from build123d import *

# Parameters (mm, degrees)
SKETCH_1_R      = 2.5
EXTRUDE_1_DEPTH = 4
FILLET_1_R      = 5


with BuildPart() as part:
    # ｽｹｯﾁ1 → ﾎﾞｽ - 押し出し1 (new body)
    with BuildSketch(Plane.XY):
        Polygon((0, 15), (0, 0), (4, 0), (4, -6), (8.110763801, -6), (24, -2.18322685), (24, 8.312378031), (4, 22), (4, 15), align=None)
        with Locations((14, 3)):
            Circle(SKETCH_1_R, mode=Mode.SUBTRACT)
    extrude(amount=EXTRUDE_1_DEPTH)

    # ﾌｨﾚｯﾄ1
    fillet_1_edges = [part.edges().sort_by_distance(p)[0] for p in [
        (24, -2.18322685, 2),
        (24, 8.312378031, 2),
    ]]
    fillet(fillet_1_edges, radius=FILLET_1_R)


solid = part.part
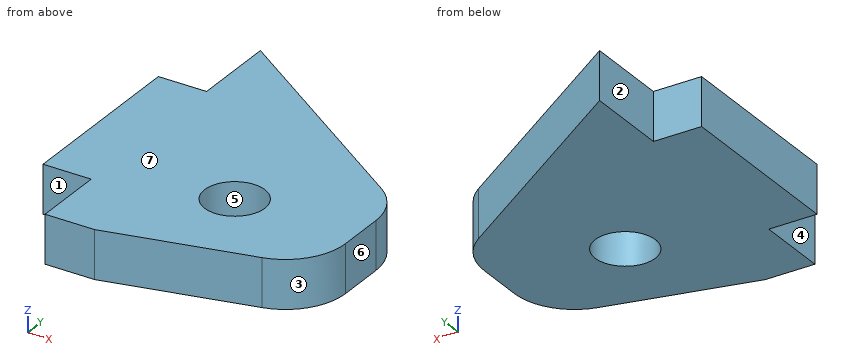
Read the model definition and answer for the solid it produces. Units are mm, in the model's axes. Face numbers are marked on the shaded views. A direction names the side the tool comes from. Give positions to 0.01 mm unless a question says otherwise; leave off trailing zeros. Write each loop counter-clockwise with the first axis right and the second up, starting at its lowest first coordinate (ties: lowest second). Pieces come first, ordered by that corner, then holes. Notation, with made-up numbers: M 2.5,7 L 47.5,7 A30 ccw 47.5,41 Z; hole C 67.25,-34.5 d11. An arc over 180 degrees is marked long. One line per item, written item: value. Start each with the question number.
(1) Find section A-A (z = 3.7). Determine the outline of the cut face in (x, y), plus the area to 3 significant figures.
(2) Find section D-D (x = 2.25). Determine the outline of the cut face in (y, z).
(3) Find section C-C (x = 13.5). Determine the outline of the cut face in (y, z).
(4) A tool of negligible diameter and unlimited length cuts with its end or side. For the marked faces 1, 2 and 3, from which of +Z, -Z, +X, -X, +Y, -Y can it reach the whole face along a straight path? Write none if from no direction.
(5) Flat-ended cylindrical pins translate along their axes: pin 1 Ø1.2 at (y, z) = (17.5, 2.5) entering from -X; pin 2 Ø3 at (x, y) = (14, 3) entering from -Z; pin 3 Ø2 at (x, z) = (8.5, 2.5) entering from +Y. Find the tip coordinate at first contact, or state that the pin passes through.
(6) Find the intervals of material crossed by line 1 (X direction, y = 2.5, z = 0.25); line 2 (X direction, y = 2.75, z = 3.5); line 3 (Y direction, x = 3.75, z = 3.55), in increasing order.
(7) Determine the mould class of the marked faces 4, 5, 6 and 7 for opening direction X: pulls with the +X half, pulls with the -X half, needs draft (parallel to the pull), parting line crosses it, or undercut.
(8) Find section B-B (y = 3). Determine the outline of the cut face in (x, z).
Results below:
1. outline: M 0,0 L 4,0 L 4,-6 L 8.11,-6 L 20.17,-3.1 A5 ccw 24,1.76 L 24,5.68 A5 ccw 21.82,9.8 L 4,22 L 4,15 L 0,15 Z; hole C 14,3 d5
1. area: 429 mm^2
2. outline: M 0,0 L 15,0 L 15,4 L 0,4 Z
3. outline: M -4.71,0 L 0.55,0 L 0.55,4 L -4.71,4 Z; M 5.45,0 L 15.5,0 L 15.5,4 L 5.45,4 Z
4. face 1: +Z, -Z, -X, -Y
4. face 2: +Z, -Z, -X, +Y
4. face 3: +Z, -Z, +X, -Y
5. pin 1: stops at x = 4
5. pin 2: passes through
5. pin 3: stops at y = 19.6
6. line 1: x = 0 to 11.55, 16.45 to 24
6. line 2: x = 0 to 11.51, 16.49 to 24
6. line 3: y = 0 to 15
7. face 4: pulls with the -X half
7. face 5: undercut
7. face 6: pulls with the +X half
7. face 7: needs draft
8. outline: M 0,0 L 11.5,0 L 11.5,4 L 0,4 Z; M 16.5,0 L 24,0 L 24,4 L 16.5,4 Z
